from build123d import *

# Parameters (mm, degrees)
F0_W     = 52
F0_H     = 74
F1_DEPTH = 10
F2_R     = 2.5
F3_DEPTH = 19
F4_R     = 1
F5_SIZE  = 2


with BuildPart() as f1:
    # F0 (on Top) → F1 (new body)
    with BuildSketch(Plane.XY):
        Rectangle(F0_W, F0_H)
    extrude(amount=F1_DEPTH)

    # F2 (on face) → F3 (join)
    with BuildSketch(Plane.XY.offset(10)):
        with Locations((0, 10)):
            Circle(F2_R)
        with Locations((0, -10)):
            Circle(F2_R)
    extrude(amount=F3_DEPTH)

    # F4
    f4_edges = [f1.edges().sort_by_distance(p)[0] for p in [
        (-2.5, 10, 29),
        (-2.5, -10, 29),
    ]]
    fillet(f4_edges, radius=F4_R)

    # F5
    f5_edges = [f1.edges().sort_by_distance(p)[0] for p in [
        (0, 37, 10),
        (26, 0, 10),
        (-26, 0, 10),
        (0, -37, 10),
        (-26, -37, 5),
        (26, -37, 5),
        (-26, 37, 5),
        (26, 37, 5),
    ]]
    chamfer(f5_edges, length=F5_SIZE)


solid = f1.part
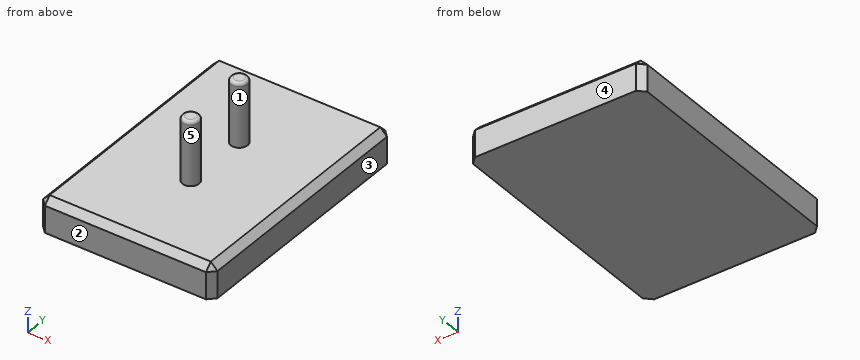
Work out the finished part from the listing and answer in its coordinate system (mm). Face numbers are marked on the shaded views. A direction names the side the tool comes from. Give positions to 0.01 mm unless a question says otherwise; leave off trailing zeros. Order: outer loops, then holes, each group sorted by start corner. A loop starts at its lowest first (then second) coordinate and runs counter-clockwise, first axis right, second up. Notation, with made-up numbers: M 75.25,65 L 84.25,65 A30 ccw 84.25,90 Z; hole C 61,-13 d4. An arc over 180 degrees is marked long. Return JSON: item names as keys, results as strings.
Q1. The mould has two halves that part along Y. Classify the marked faces 1, 2 and 3: pulls with the +Y half, pulls with the -Y half, needs draft (parallel to the pull), parting line crosses it, or undercut.
Answer below:
{"face 1": "undercut", "face 2": "pulls with the -Y half", "face 3": "needs draft"}
Q2. Find section D-D, the plane y = 19. Write down the section's boundary in (x, z), and give its area (3 significant figures).
Answer below:
{"outline": "M -26,0 L 26,0 L 26,8 L 24,10 L -24,10 L -26,8 Z", "area": "516 mm^2"}
Q3. Find the intervals of material crossed by line 1 along Y through (x, z) = (0, 19.25); line 2 along Z through (x, y) = (-15.5, -19.5); line 3 along X through (y, z) = (-8, 22.5), in increasing order. Write a range as [from, to].
Answer below:
{"line 1": "y = [-12.5, -7.5], [7.5, 12.5]", "line 2": "z = [0, 10]", "line 3": "x = [-1.5, 1.5]"}
Q4. This flat-tipped pin is pushed along its axis until it touches: pin 1 (12 mm diameter, centred on x = -15, y = -18.5, fed in from +Z). Where does it stop, or does it pass through?
Answer below:
{"pin 1": "stops at z = 10"}
Q5. Which of the six approach directions +Z, -Z, +X, -X, +Y, -Y give full straight-line access (tool end or side, diameter ignored) to the marked faces 4 and 5?
Answer below:
{"face 4": "+Z, -Z, +X, -X, +Y", "face 5": "+Z"}
Q6. Find section C-C, the plane z = 21.5. Write down the section's boundary in (x, y).
Answer below:
{"outline": "C 0,-10 d5; C 0,10 d5"}
Q7. Find section A-A, the plane y = -10. Write down the section's boundary in (x, z), and give its area (3 significant figures).
Answer below:
{"outline": "M -26,0 L 26,0 L 26,8 L 24,10 L 2.5,10 L 2.5,28 A1 ccw 1.5,29 L -1.5,29 A1 ccw -2.5,28 L -2.5,10 L -24,10 L -26,8 Z", "area": "611 mm^2"}
Q8. Find section B-B, the plane x = 0. Write down the section's boundary in (y, z).
Answer below:
{"outline": "M -37,0 L 37,0 L 37,8 L 35,10 L 12.5,10 L 12.5,28 A1 ccw 11.5,29 L 8.5,29 A1 ccw 7.5,28 L 7.5,10 L -7.5,10 L -7.5,28 A1 ccw -8.5,29 L -11.5,29 A1 ccw -12.5,28 L -12.5,10 L -35,10 L -37,8 Z"}
